from build123d import *

# Parameters (mm, degrees)
F0_W     = 55
F0_H     = 12
F1_DEPTH = 6
F2_R     = 2.5
F3_DEPTH = 12.001
F5_DEPTH = 25


with BuildPart() as f1:
    # F0 (on Top) → F1 (new body, symmetric)
    with BuildSketch(Plane.XY):
        Rectangle(F0_W, F0_H)
    extrude(amount=F1_DEPTH, both=True)

    # F2 (on face) → F3 (cut, through all)
    with BuildSketch(Plane.XY.offset(6)):
        with Locations((-19.5, 0)):
            Circle(F2_R)
        with Locations((19.5, 0)):
            Circle(F2_R)
    extrude(amount=-F3_DEPTH, mode=Mode.SUBTRACT)

    # F4 (on face) → F5 (cut)
    with BuildSketch(Plane.XZ.offset(6)):
        with BuildLine():
            ThreePointArc((0.006891, 2.291288), (-10.493109, 0), (0.006891, -2.291288))
            ThreePointArc((0.006891, -2.291288), (10.506891, 0), (0.006891, 2.291288))
        make_face()
    extrude(amount=-F5_DEPTH, mode=Mode.SUBTRACT)


solid = f1.part
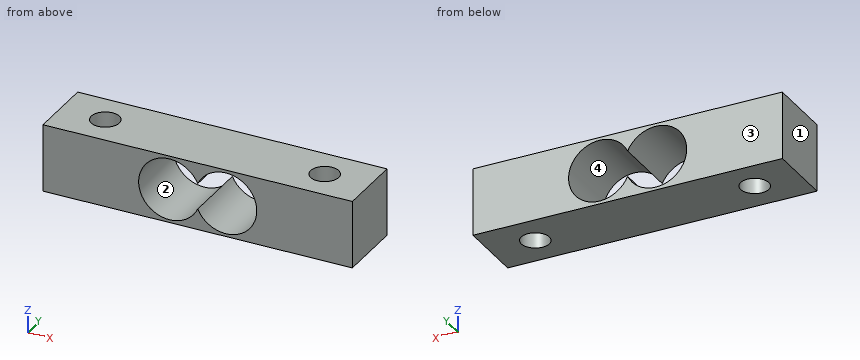
Verification items for the finished model (mm, model axes). Face numbers are marked on the shaded views. Coordinates: 2 decimals unless noted, no trailing zeros. Order: outer loops, then holes, each group sorted by start corner. A loop starts at its lowest first (then second) coordinate and runs counter-clockwise, first axis right, second up. Notation, with made-up numbers: M 55,-2 L 69,-2 A21 cw 69,30 Z; hole C 5.25,62.5 d10. An arc over 180 degrees is marked long. One line per item, written item: value. Start each with the question number.
Item 1: Sectioned sample at C-C (x = -19.5). Enter the section's corners in (y, z), then the cut area to 3 significant figures.
Item 2: Sectioned sample at A-A (y = 0.5). Enter the section's corners in (x, z), then the cut area to 3 significant figures.
Item 3: Sectioned sample at B-B (z = 0). Enter the section's corners in (x, y).
Item 4: Scan lines: probe 1 along Y at (x, z) = (19.5, 2.25); probe 2 along X at (y, z) = (-0.5, 0); probe 3 along X at (y, z) = (-5, 4). Record each from-to range of solid material in increasing order.
Item 5: Mould release check, pull along X, two halves, no side actions. Record for the marked faces 1, 2, 3 and 4: released by +X, released by -X, zero draft, split by the parting line, or undercut.
Item 6: Gauge pin test, flat end, axial feed: pin 1 (6.5 mm diameter, centred on x = 5.01, z = 0, fed in from -Y). Record the tip position at first contact, or that the pin passes through.
Item 7: Sectioned sample at D-D (z = 4.5). Enter the section's corners in (x, y).
Conclusion:
1. outline: M -6,-6 L -2.5,-6 L -2.5,6 L -6,6 Z; M 2.5,-6 L 6,-6 L 6,6 L 2.5,6 Z
1. area: 84.0 mm^2
2. outline: M -27.5,-6 L -21.95,-6 L -21.95,6 L -27.5,6 Z; M -17.05,-6 L 17.05,-6 L 17.05,6 L -17.05,6 Z; M 21.95,-6 L 27.5,-6 L 27.5,6 L 21.95,6 Z; hole M 0.01,-2.29 A5.5 ccw long 0.01,2.29 A5.5 ccw long Z
2. area: 355 mm^2
3. outline: M -27.5,-6 L -10.49,-6 L -10.49,6 L -27.5,6 Z; M 10.51,-6 L 27.5,-6 L 27.5,6 L 10.51,6 Z; hole C -19.5,0 d5; hole C 19.5,0 d5
4. probe 1: y = -6 to -2.5, 2.5 to 6
4. probe 2: x = -27.5 to -21.95, -17.05 to -10.49, 10.51 to 17.05, 21.95 to 27.5
4. probe 3: x = -27.5 to -8.77, -1.22 to 1.23, 8.78 to 27.5
5. face 1: released by -X
5. face 2: undercut
5. face 3: zero draft
5. face 4: undercut
6. pin 1: passes through
7. outline: M -27.5,-6 L -8.16,-6 L -8.16,6 L -27.5,6 Z; M -1.83,-6 L 1.84,-6 L 1.84,6 L -1.83,6 Z; M 8.17,-6 L 27.5,-6 L 27.5,6 L 8.17,6 Z; hole C -19.5,0 d5; hole C 19.5,0 d5
